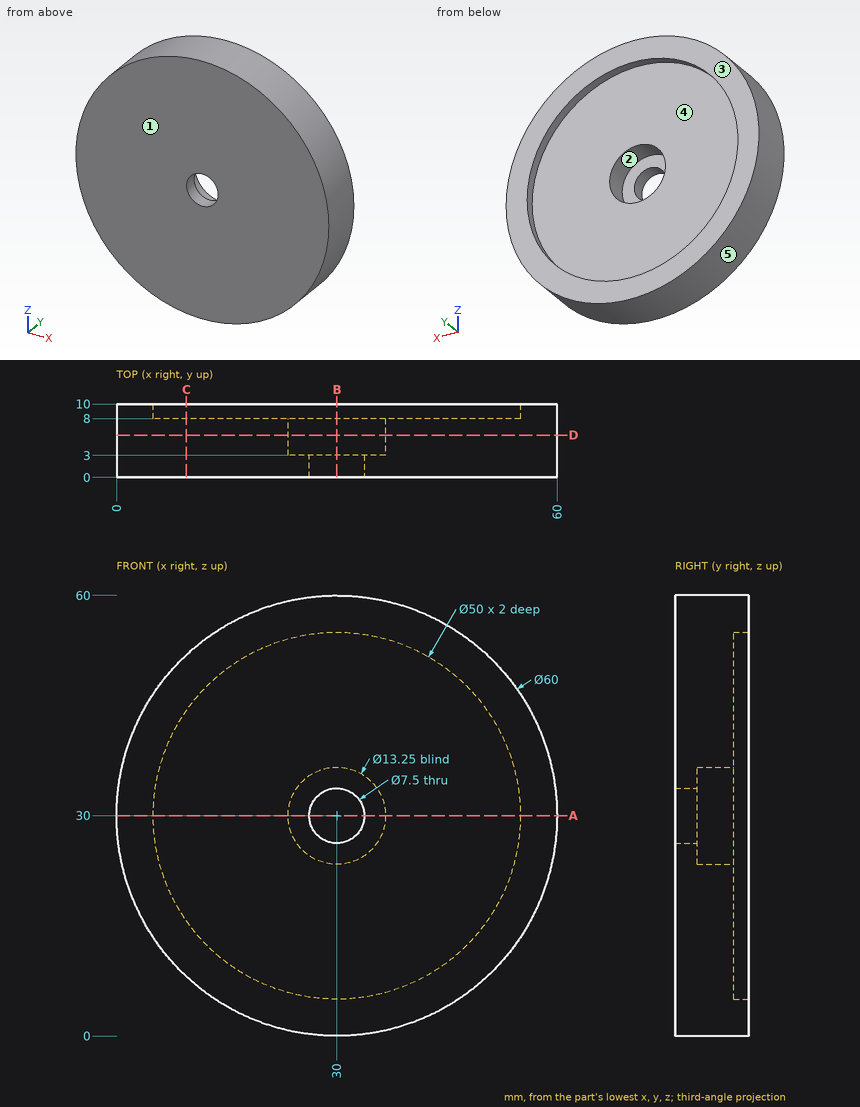
Can you work these out from the drawing? Everything is in mm from the part's minimum corner. A direction names the side the tool comes from. Coordinates: 2 decimals unless noted, no trailing zeros. Write each loop counter-clockwise with the first axis right and the second up, starting at its lowest first coordinate (ties: lowest second). Pieces come first, ordered by that corner, then holes. Notation, with made-up numbers: (-5, 73.25) -> (46, 73.25) arc R19 cw to (46, 82.25) -> close; hole circle Ø9 at (-38, 12.5). An arc over 180 degrees is marked (long way). Write each question's results on one line, items separated by ' | '. Start each with the question number.
Item 1: If we section it at C-C, the plane x = 9.5: Write out the boundary of the cut face in (y, z).
Item 2: If we section it at B-B, the plane x = 30: Write out the boundary of the cut face in (y, z) (3 decimals).
Item 3: Please list where these lines run through material, in increasing order: probe 1 along Z at (x, y) = (30, 1.95); probe 2 along X at (y, z) = (9.05, 30); probe 3 along Z at (x, y) = (30, 4.7) (3 decimals).
Item 4: I'm going to push flat-ended pins straight in: P1, Ø10, axis at x = 47, z = 32, coming from the -Y side; P2, Ø4, axis at x = 30, z = 32, coming from the +Y side; P3, Ø2, axis at y = 4, z = 16.5, coming from the -X side; P4, Ø12, axis at x = 38, z = 18, coming from the +Y side. Where does each tip first touch, or does it pass through?
Item 5: Thinking about a two-plate mould opening in X: for the marked faces 3, 4 and 5, which applies, released by +X, released by -X, zero draft, split by the parting line, or undercut?
Item 6: If we section it at D-D, the plane y = 5.75: Write out the boundary of the cut face in (x, z) (3 decimals).
Item 7: If we section it at A-A, the plane z = 30: Write out the boundary of the cut face in (x, y) (3 decimals).
Item 8: On a 3-axis mill with a long thin cutter (end or side, diameter ignored), from which of +Z, -Z, +X, -X, +Y, -Y can I reach the whole of each face in a straight line? I mean the marked faces 1 and 2. Say none if no direction works.
Answer block:
1) outline: (0, 8.1) -> (10, 8.1) -> (10, 15.69) -> (8, 15.69) -> (8, 44.31) -> (10, 44.31) -> (10, 51.9) -> (0, 51.9) -> close
2) outline: (0, 0) -> (10, 0) -> (10, 5) -> (8, 5) -> (8, 23.375) -> (3, 23.375) -> (3, 26.25) -> (0, 26.25) -> close; (0, 33.75) -> (3, 33.75) -> (3, 36.625) -> (8, 36.625) -> (8, 55) -> (10, 55) -> (10, 60) -> (0, 60) -> close
3) probe 1: 0 to 26.25, 33.75 to 60 | probe 2: 0 to 5, 55 to 60 | probe 3: 0 to 23.375, 36.625 to 60
4) P1: y = 0 | P2: y = 3 | P3: x = 2.73 | P4: y = 8
5) face 3: zero draft | face 4: undercut | face 5: split by the parting line
6) outline: circle Ø60 at (30, 30); hole circle Ø13.25 at (30, 30)
7) outline: (0, 0) -> (26.25, 0) -> (26.25, 3) -> (23.375, 3) -> (23.375, 8) -> (5, 8) -> (5, 10) -> (0, 10) -> close; (33.75, 0) -> (60, 0) -> (60, 10) -> (55, 10) -> (55, 8) -> (36.625, 8) -> (36.625, 3) -> (33.75, 3) -> close
8) face 1: +Z, -Z, +X, -X, -Y | face 2: +Y
